Solid Edge part; units mm, degrees
sketch "Sketch1" plane through (0, 0, 0) normal (0, 0, 1) x (1, 0, 0)
  line L0 (-18, -18) -> (18, -18)
  line L1 (18, -18) -> (18, 18)
  line L2 (18, 18) -> (-18, 18)
  line L3 (-18, 18) -> (-18, -18)
  dimension "D1" = 18
extrude "Protrusion1" add sketch "Sketch1" along normal blind 3
sketch "Sketch2" plane through (0, 0, 3) normal (0, 0, 1) x (1, 0, 0)
  circle A0 centre (13, 13) radius 1
  circle A1 centre (13, -13) radius 1
  circle A2 centre (-13, -13) radius 1
  circle A3 centre (-13, 13) radius 1
extrude "Cutout1" cut sketch "Sketch2" against normal up to next
sketch "Sketch3" plane through (0, 0, 3) normal (0, 0, 1) x (0, 1, 0)
  line L0 (-8, 12) -> (0, 12)
  line L1 (0, 12) -> (0, 17)
  line L2 (0, 17) -> (-8, 17)
  line L3 (-8, 17) -> (-8, 12)
extrude "Collegamento_cavi" add sketch "Sketch3" along normal blind 5
sketch "Sketch4" plane through (0, 0, 3) normal (0, 0, 1) x (0, 1, 0)
  line L0 (6.5, 12.5) -> (10.5, 12.5)
  line L1 (10.5, 12.5) -> (10.5, 16.5)
  line L2 (10.5, 16.5) -> (6.5, 16.5)
  line L3 (6.5, 16.5) -> (6.5, 12.5)
extrude "Collegamento_secondario" add sketch "Sketch4" along normal blind 3
sketch "Sketch5" plane through (0, 0, 3) normal (0, 0, 1) x (0, 1, 0)
  line L0 (-2.5, 4) -> (-10.5, 4)
  line L1 (-10.5, 4) -> (-10.5, -4)
  line L2 (-10.5, -4) -> (-2.5, -4)
  line L3 (-2.5, -4) -> (-2.5, 4)
extrude "Scheda" add sketch "Sketch5" along normal blind 1
sketch "Sketch6" plane through (0, 0, 3) normal (0, 0, 1) x (0, 1, 0)
  line L0 (1, 2.5) -> (1, -2.5)
  line L1 (1, -2.5) -> (6, -2.5)
  line L2 (6, -2.5) -> (6, 2.5)
  line L3 (6, 2.5) -> (1, 2.5)
extrude "Schedina" add sketch "Sketch6" along normal blind 1
sketch "Sketch7" plane through (0, 0, 3) normal (0, 0, 1) x (0, 1, 0)
  circle A0 centre (6, -10) radius 2.5
extrude "Protrusione_circolare" add sketch "Sketch7" along normal blind 1
sketch "Sketch8" plane through (0, 0, 3) normal (0, 0, 1) x (0, 1, 0)
  line L0 (9, -4) -> (17, -4)
  line L1 (17, -4) -> (17, 4)
  line L2 (17, 4) -> (9, 4)
  line L3 (9, 4) -> (9, -4)
extrude "Collegamento_Camera" add sketch "Sketch8" along normal blind 2
sketch "Sketch9" plane through (0, 0, 3) normal (0, 0, 1) x (0, 1, 0)
  line L0 (-4, -16) -> (-4, -12)
  line L1 (-4, -12) -> (-8, -12)
  line L2 (-8, -12) -> (-8, -16)
  line L3 (-8, -16) -> (-4, -16)
extrude "Scheda_laterale" add sketch "Sketch9" along normal blind 1
sketch "Sketch10" plane through (0, 0, 3) normal (0, 0, 1) x (0, 1, 0)
  line L0 (16.5, 9) -> (12.5, 9)
  line L1 (12.5, 9) -> (12.5, 5)
  line L2 (12.5, 5) -> (16.5, 5)
  line L3 (16.5, 5) -> (16.5, 9)
extrude "Scheda_posteriore" add sketch "Sketch10" along normal blind 1
fillet "Rotondo_1" radius 5 4 edges at (18, -18, 1.5) (18, 18, 1.5) (-18, -18, 1.5) (-18, 18, 1.5)
sketch "Sketch11" plane through (0, 13, 5) normal (0, 0, 1) x (-1, 0, 0)
  line L0 (-2, -4) -> (2, -4)
  line L1 (2, -4) -> (2, 1.5)
  line L2 (2, 1.5) -> (-2, 1.5)
  line L3 (-2, 1.5) -> (-2, -4)
  dimension "D1" = 2
  dimension "D2" = 2
extrude "Alloggio_cavi_Camera" cut sketch "Sketch11" against normal blind 1
sketch "Sketch12" plane through (0, 0, 3) normal (0, 0, 1) x (-1, 0, 0)
  line L0 (5, 13) -> (-5, 13)
  line L1 (-5, 13) -> (-5, 16)
  line L2 (-5, 16) -> (5, 16)
  line L3 (5, 16) -> (5, 13)
extrude "ProtrusioneEstrusa_12" add sketch "Sketch12" along normal blind 2
sketch "Sketch13" plane through (0, 14.25, 4) normal (0, 0, 1) x (-1, 0, 0)
  line L0 (-0.8, -2.75) -> (-0.8, 1.25)
  line L1 (-0.8, 1.25) -> (-0.6, 1.25)
  line L2 (-0.6, 1.25) -> (-0.6, -2.75)
  line L3 (-0.6, -2.75) -> (-0.8, -2.75)
  line L4 (0.1, 1.25) -> (0.1, -2.75)
  line L5 (0.1, -2.75) -> (-0.1, -2.75)
  line L6 (-0.1, -2.75) -> (-0.1, 1.25)
  line L7 (-0.1, 1.25) -> (0.1, 1.25)
  line L8 (0.8, -2.75) -> (0.8, 1.25)
  line L9 (0.8, 1.25) -> (0.6, 1.25)
  line L10 (0.6, 1.25) -> (0.6, -2.75)
  line L11 (0.6, -2.75) -> (0.8, -2.75)
extrude "ProtrusioneEstrusa_13" add sketch "Sketch13" along normal blind 0.1
The listing builds one solid part. Answer for the finished solid, in the listing's coordinates (mm). A direction names the side the tool comes from. Give positions to 0.01 mm unless a question says otherwise; leave off trailing zeros. Order: outer loops, then holes, each group sorted by start corner. A loop starts at its lowest first (then second) coordinate and runs counter-clockwise, first axis right, second up. Notation, with made-up numbers: (8.5, -18.5) - (42.5, -18.5) arc R25 ccw to (42.5, 20.5) - close; hole circle Ø6 at (-29, 57.25). An arc over 180 degrees is marked (long way). Use one line per item in the form item = value. Start each with the question number.
(1) Flat-ended cylindrical pins translate along their axes: pin 1 Ø0.9 at (x, z) = (-15, 4.5) entering from +Y; pin 2 Ø3 at (x, y) = (14.5, -5.5) entering from +Z; pin 3 Ø0.5 at (x, z) = (0, 4.5) entering from +Y; pin 4 Ø1.6 at (x, y) = (-13, 13) entering from -Z. Find the tip coordinate at first contact, or state that the pin passes through.
(2) Consider line 1 (Y direction, x = -13, z = 1.6); line 2 (X direction, y = 11.5, z = 3.25); line 3 (Z direction, x = 8.5, y = 12). Determine where each line is inside the solid, lowest interval first. Write a range as from..to.
(3) A cutting plane is placed at C-C, the plane z = 3.5. State how many separate pieces and enclosed holes the cut face has, then the cut area to 3 significant figures.
(4) A cutting plane is placed at D-D, the plane x = 3. Write down the section's boundary in (y, z).
(5) The mould has two halves that part along X. Classify faces 4 (the flat face through (14, -6, 4)), 5 (the flat face through (16, -6, 3.5)), 6 (the flat face through (-4, 13, 4)): released by +X, released by -X, zero draft, split by the parting line, or undercut.
(6) A cutting plane is placed at A-A, the plane y = -5. Write down the section's boundary in (x, z).
(7) For faces 1 (the flat face through (0, 9, 4)), 2 (the flat face through (0, -16, 4)), 3 (the flat face through (0, 11, 5)), determine the directions among +Z, -Z, +X, -X, +Y, -Y from which every point of the face is accessible in a straight line to the end or side of a thin tool.
(8) A cutting plane is placed at B-B, the plane x = 10. Write down the section's boundary in (y, z).
Ans:
q1.pin_1 = 10.5
q1.pin_2 = 4
q1.pin_3 = 11.5
q1.pin_4 = through
q2.line_1 = -18..-14, -12..12, 14..18
q2.line_2 = -4..4
q2.line_3 = 0..3
q3.separate_pieces = 9
q3.enclosed_holes = 0
q3.area = 291 mm^2
q4.outline = (-18, 0) - (18, 0) - (18, 3) - (17, 3) - (17, 5) - (9, 5) - (9, 3) - (-2.5, 3) - (-2.5, 4) - (-10.5, 4) - (-10.5, 3) - (-13, 3) - (-13, 5) - (-16, 5) - (-16, 3) - (-18, 3) - close
q5.face_4 = zero draft
q5.face_5 = released by +X
q5.face_6 = undercut
q6.outline = (-18, 0) - (18, 0) - (18, 3) - (16, 3) - (16, 4) - (12, 4) - (12, 3) - (4, 3) - (4, 4) - (-4, 4) - (-4, 3) - (-12, 3) - (-12, 8) - (-17, 8) - (-17, 3) - (-18, 3) - close
q7.face_1 = +Z, +X
q7.face_2 = +Z, +X, -X, -Y
q7.face_3 = +Z, +X, +Y, -Y
q8.outline = (-18, 0) - (18, 0) - (18, 3) - (8.5, 3) - (8.5, 4) - (3.5, 4) - (3.5, 3) - (-18, 3) - close
